```python
from build123d import *

# Parameters (mm, degrees)
SKETCH_1_W          = 12.1
SKETCH_1_H          = 22.5
EXTRUDE_1_DEPTH     = 20
SKETCH_2_W          = 12.1
SKETCH_2_H          = 2
EXTRUDE_2_DEPTH     = 4.8
SKETCH_3_W          = 12.1
SKETCH_3_H          = 2
EXTRUDE_3_DEPTH     = 4.8
SKETCH_4_R          = 0.625
CUT_EXTRUDE_1_DEPTH = 35.843819526
EXTRUDE_4_DEPTH     = 4
SKETCH_6_R          = 2.239241923
EXTRUDE_5_DEPTH     = 3
SKETCH_7_W          = 3.584102009
SKETCH_7_H          = 0.896025503
EXTRUDE_6_DEPTH     = 3


with BuildPart() as part:
    # 草图1 → 凸台-拉伸1 (new body)
    with BuildSketch(Plane(origin=(0, 0, 0), x_dir=(1, 0, 0), z_dir=(0, 1, 0))):
        with Locations((5.726041667, -11.361979167)):
            Rectangle(SKETCH_1_W, SKETCH_1_H)
    extrude(amount=EXTRUDE_1_DEPTH)

    # 草图2 → 凸台-拉伸2 (add)
    with BuildSketch(Plane.XY.offset(22.611979167)):
        with Locations((5.726041667, 17)):
            Rectangle(SKETCH_2_W, SKETCH_2_H)
    extrude(amount=EXTRUDE_2_DEPTH)

    # 草图3 → 凸台-拉伸3 (add)
    with BuildSketch(Plane(origin=(0, 0, 0.111979167), x_dir=(-1, 0, 0), z_dir=(0, 0, -1))):
        with Locations((-5.726041667, 17)):
            Rectangle(SKETCH_3_W, SKETCH_3_H)
    extrude(amount=EXTRUDE_3_DEPTH)

    # 草图4 → 切除-拉伸1 (cut, through all)
    with BuildSketch(Plane(origin=(0, 18, 0), x_dir=(1, 0, 0), z_dir=(0, 1, 0))):
        with Locations(Location((5.726041667, 2.288020833, 0), (0, 0, 270))):
            Circle(SKETCH_4_R)
        with Locations(Location((5.726041667, -25.011979167, 0), (0, 0, 270))):
            Circle(SKETCH_4_R)
    extrude(amount=-CUT_EXTRUDE_1_DEPTH, mode=Mode.SUBTRACT)

    # 草图5 → 凸台-拉伸4 (add)
    with BuildSketch(Plane(origin=(0, 20, 0), x_dir=(1, 0, 0), z_dir=(0, 1, 0))):
        with BuildLine():
            Line((8.226041667, -4.676017513), (8.226041667, -10.900780437))
            ThreePointArc((8.226041667, -10.900780437), (5.726041667, -22.460090739), (3.226041667, -10.900780437))
            Line((3.226041667, -10.900780437), (3.226041667, -4.676017412))
            ThreePointArc((3.226041667, -4.676017412), (5.726041717, -2.176017463), (8.226041667, -4.676017513))
        make_face()
    extrude(amount=EXTRUDE_4_DEPTH)

    # 草图6 → 凸台-拉伸5 (add)
    with BuildSketch(Plane(origin=(0, 24, 0), x_dir=(1, 0, 0), z_dir=(0, 1, 0))):
        with Locations(Location((5.726041667, -16.410090739, 0), (0, 0, 270))):
            Circle(SKETCH_6_R)
    extrude(amount=EXTRUDE_5_DEPTH)

    # 草图7 → 凸台-拉伸6 (add)
    with BuildSketch(Plane.XY.offset(22.611979167)):
        with Locations((5.726041667, 2.764925233)):
            Rectangle(SKETCH_7_W, SKETCH_7_H)
    extrude(amount=EXTRUDE_6_DEPTH)


solid = part.part
```
Geometry: final body of the model. Coordinates: model frame, mm. A direction names the side the tool comes from. Coordinates: 2 decimals unless noted, no trailing zeros. Loops run counter-clockwise (first coordinate to the right, second up) from the corner with the lowest first, then second, coordinate; pieces in that order, holes last. Notation, with made-up numbers: M -21,-28 L 38,-28 A37 ccw 38,10 Z; hole C -38.5,22.25 d11. An arc over 180 degrees is marked long. Put each result on its own line as item: value.
(1) Draft query along Y for faces 1 (the face through (3.226, 22, 8)), 2 (the face through (6, 3.213, 24)), 3 (the face through (5.8, 18, -3.3)). Return one class per face: pulls with the +Y half, pulls with the -Y half, needs draft (parallel to the pull), parting line crosses it, or undercut.
Answer sheet:
face 1: needs draft
face 2: undercut
face 3: pulls with the +Y half
(2) First-contact query: pin 1 (4 mm diameter, centred on x = 7.5, z = 26, fed in from -Y); pin 2 (1.5 mm diameter, centred on x = 6.5, z = 24, fed in from +Y); pin 3 (2.5 mm diameter, centred on x = 8.5, z = -2, fed in from -Y); pin 4 (0.8 mm diameter, centred on x = 5.73, z = -2.29, fed in from +Y). Flat tips, straight axial feed; report the tip coordinate or a pass-through.
Answer sheet:
pin 1: stops at y = 2.32
pin 2: stops at y = 18
pin 3: stops at y = 16
pin 4: passes through
(3) Cut plane D-D on z = 19. Return the cut outline in (x, y), then the cut area to 3 significant figures.
Answer sheet:
outline: M -0.32,0 L 11.78,0 L 11.78,20 L 11.19,20 L 11.19,24 L 0.26,24 L 0.26,20 L -0.32,20 Z
area: 286 mm^2
(4) Access query for faces 4 (the face through (6.399, 25.479, 18.546)), 5 (the face through (6, 19, 0.112)), 6 (the face through (6, 16, 26)). Directions: +Z, -Z, +X, -X, +Y, -Y. A direction counts if a zero-diameter tool reaches every point of the face in a straight line with its end or side. Return the directions, or none.
Answer sheet:
face 4: +Y
face 5: -Z, +X, -X, +Y
face 6: +Z, +X, -X
(5) Cut plane A-A on z = 7. Return the cut outline in (x, y), then the cut area to 3 significant figures.
Answer sheet:
outline: M -0.32,0 L 11.78,0 L 11.78,20 L 8.23,20 L 8.23,24 L 3.23,24 L 3.23,20 L -0.32,20 Z
area: 262 mm^2
(6) Cut plane B-B on x = 10.5. Return the cut outline in (y, z), then the cut area to 3 significant figures.
Answer sheet:
outline: M 0,0.11 L 16,0.11 L 16,-4.69 L 18,-4.69 L 18,0.11 L 20,0.11 L 20,12.69 L 24,12.69 L 24,20.13 L 20,20.13 L 20,22.61 L 18,22.61 L 18,27.41 L 16,27.41 L 16,22.61 L 0,22.61 Z
area: 499 mm^2
(7) Cut plane C-C on y = 7.5. Return the cut outline in (x, z).
Answer sheet:
outline: M -0.32,0.11 L 11.78,0.11 L 11.78,22.61 L -0.32,22.61 Z
(8) Material intervals for probe 1 along Z at (x, y) = (10.75, 15.5); probe 2 along Y at (x, z) = (1, 23.5); probe 3 along Y at (x, z) = (1.5, 16.5), sorted ascending.
Answer sheet:
probe 1: z = 0.11 to 22.61
probe 2: y = 16 to 18
probe 3: y = 0 to 24
